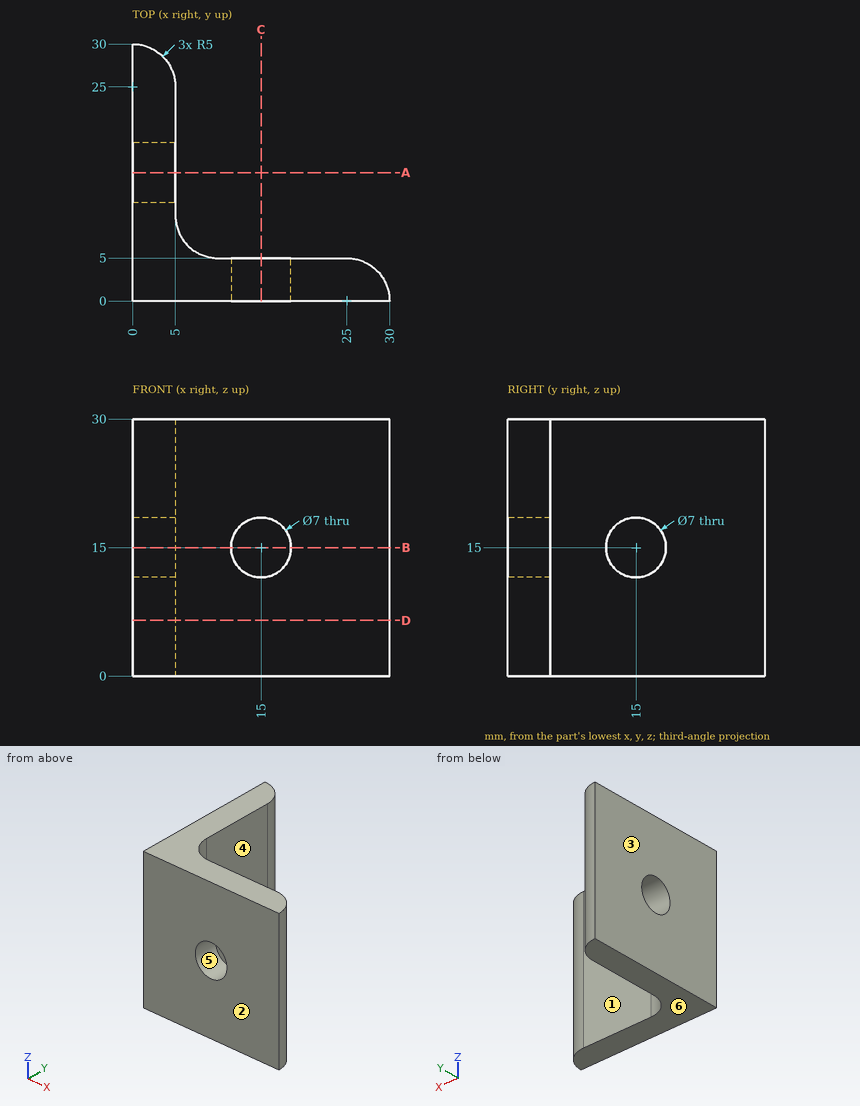
Source: three-view drawing plus pictorial views. Frame: mm from the lowest corner of the part. A direction names the side the tool comes from. Round coordinates to 2 decimals unless told otherwise and drop trailing zeros. Write each loop counter-clockwise with the first axis right and the second up, starting at its lowest first coordinate (ties: lowest second). Pieces come first, ordered by that corner, then holes. Notation, with made-up numbers: M 21,-36 L 27,-36 A16 ccw 27,-17 Z; hole C -4,51 d4. An arc over 180 degrees is marked long. Write each question's results on one line, items separated by ' | '.
Q1. Section query D-D (z = 6.5). Return loops of the section in (x, y), and give its area (3 significant figures).
Results:
outline: M 0,0 L 30,0 A5 ccw 25,5 L 10,5 A5 cw 5,10 L 5,25 A5 ccw 0,30 Z | area: 270 mm^2
Q2. Access query for the marked faces 1 and 2. Directions: +Z, -Z, +X, -X, +Y, -Y. A direction counts if a zero-diameter tool reaches every point of the face in a straight line with its end or side. Return the directions, or none.
Results:
face 1: +Z, -Z, +X, +Y | face 2: +Z, -Z, +X, -X, -Y
Q3. Section query B-B (z = 15). Return loops of the section in (x, y).
Results:
outline: M 0,0 L 11.5,0 L 11.5,5 L 10,5 A5 cw 5,10 L 5,11.5 L 0,11.5 Z; M 0,18.5 L 5,18.5 L 5,25 A5 ccw 0,30 Z; M 18.5,0 L 30,0 A5 ccw 25,5 L 18.5,5 Z
Q4. Pin query (flat end, axial travel): P1, Ø7.5, axis at x = 18.5, z = 9.5, coming from the +Y side; P2, Ø7.5, axis at y = 19.5, z = 13.5, coming from the +X side; P3, Ø2, axis at x = 9, z = 20, coming from the +Y side; P4, Ø4, axis at x = 12, y = 7.5, coming from the +Z side (1 decimal). Return the tip coordinate at first contact, or that it passes through.
Results:
P1: stops at y = 5 | P2: stops at x = 5 | P3: stops at y = 5.42 | P4: passes through
Q5. Draft query along X for the marked faces 3, 4, 5 and 6. Return one class per face: released by +X, released by -X, zero draft, split by the parting line, or undercut.
Results:
face 3: released by -X | face 4: released by +X | face 5: undercut | face 6: zero draft
Q6. Line query: line 1 along Z through (x, y) = (2.05, 15); line 2 along X through (y, z) = (9.75, 3.75); line 3 along Y through (x, z) = (13.5, 22.5). Output: solid intervals per line, ascending.
Results:
line 1: z = 0 to 11.5, 18.5 to 30 | line 2: x = 0 to 5.01 | line 3: y = 0 to 5
Q7. Section query A-A (y = 15). Return loops of the section in (x, z), and give its area (3 significant figures).
Results:
outline: M 0,0 L 5,0 L 5,11.5 L 0,11.5 Z; M 0,18.5 L 5,18.5 L 5,30 L 0,30 Z | area: 115 mm^2
